```python
from build123d import *

# Parameters (mm, degrees)
SKETCH1_W           = 20
SKETCH1_H           = 40
BOSS_EXTRUDE1_DEPTH = 3
SKETCH4_W           = 8
SKETCH4_H           = 2.4
BOSS_EXTRUDE2_DEPTH = 20
CUT_EXTRUDE1_REACH  = 40.734
SKETCH5_R           = 1.178679728
SKETCH6_R           = 1.5
CUT_EXTRUDE2_DEPTH  = 3


with BuildPart() as part:
    # Sketch1 → Boss-Extrude1 (new body)
    with BuildSketch(Plane(origin=(0, 0, 0), x_dir=(1, 0, 0), z_dir=(0, 1, 0))):
        Rectangle(SKETCH1_W, SKETCH1_H)
    extrude(amount=BOSS_EXTRUDE1_DEPTH)

    # Sketch2 → Loft3 section 0
    with BuildSketch(Plane(origin=(0, 3, 0), x_dir=(1, 0, 0), z_dir=(0, 1, 0))):
        with BuildLine():
            Line((-10, 7.65), (10, 7.65))
            Line((10, 7.65), (10, 1.25))
            Line((10, 1.25), (-10, 1.25))
            Line((-10, 1.25), (-10, 7.65))
        make_face()
    # Sketch3 → Loft3 section 1
    with BuildSketch(Plane(origin=(0, 9, 0), x_dir=(1, 0, 0), z_dir=(0, 1, 0))):
        with BuildLine():
            Line((-4, 3.65), (4, 3.65))
            Line((4, 3.65), (4, 1.25))
            Line((4, 1.25), (-4, 1.25))
            Line((-4, 1.25), (-4, 3.65))
        make_face()
    loft3 = loft()

    # Mirror1: Loft3 across plane
    add(loft3.mirror(Plane(origin=(0, 0, 0), x_dir=(1, 0, 0), z_dir=(0, 0, -1))))

    # Sketch4 → Boss-Extrude2 (add)
    with BuildSketch(Plane(origin=(0, 9, 0), x_dir=(1, 0, 0), z_dir=(0, 1, 0))):
        with Locations((0, 2.45)):
            Rectangle(SKETCH4_W, SKETCH4_H)
        with Locations((0, -2.45)):
            Rectangle(SKETCH4_W, SKETCH4_H)
    extrude(amount=BOSS_EXTRUDE2_DEPTH)

    # Cut-Extrude1: up to this face of the body (flat: up to its plane)
    cut_extrude1_end = Plane(part.part.faces().sort_by_distance((0, 19, -3.65))[0])
    # Sketch5 → Cut-Extrude1 (cut, up to the picked face)
    with BuildSketch(Plane.XY.offset(3.65), mode=Mode.PRIVATE) as cut_extrude1_sk1:
        with BuildLine():
            Line((-4, 29), (-4, 25))
            ThreePointArc((-4, 25), (-2.828427125, 27.828427125), (0, 29))
            Line((0, 29), (-4, 29))
        make_face()
    cut_extrude1_tool1 = split(extrude(cut_extrude1_sk1.sketch, amount=-CUT_EXTRUDE1_REACH, mode=Mode.PRIVATE), bisect_by=cut_extrude1_end, keep=Keep.BOTH, mode=Mode.PRIVATE)
    # Sketch5 → Cut-Extrude1 (cut, up to the picked face)
    with BuildSketch(Plane.XY.offset(3.65), mode=Mode.PRIVATE) as cut_extrude1_sk2:
        with BuildLine():
            Line((4, 29), (0, 29))
            ThreePointArc((0, 29), (2.828427125, 27.828427125), (4, 25))
            Line((4, 25), (4, 29))
        make_face()
    cut_extrude1_tool2 = split(extrude(cut_extrude1_sk2.sketch, amount=-CUT_EXTRUDE1_REACH, mode=Mode.PRIVATE), bisect_by=cut_extrude1_end, keep=Keep.BOTH, mode=Mode.PRIVATE)
    # Sketch5 → Cut-Extrude1 (cut, up to the picked face)
    with BuildSketch(Plane.XY.offset(3.65), mode=Mode.PRIVATE) as cut_extrude1_sk3:
        with Locations((0, 25)):
            Circle(SKETCH5_R)
    cut_extrude1_tool3 = split(extrude(cut_extrude1_sk3.sketch, amount=-CUT_EXTRUDE1_REACH, mode=Mode.PRIVATE), bisect_by=cut_extrude1_end, keep=Keep.BOTH, mode=Mode.PRIVATE)
    add(cut_extrude1_tool1.solids().sort_by(Axis((-3.106528, 28.106528, 3.65), (0, 0, -1)))[0], mode=Mode.SUBTRACT)
    add(cut_extrude1_tool2.solids().sort_by(Axis((3.106528, 28.106528, 3.65), (0, 0, -1)))[0], mode=Mode.SUBTRACT)
    add(cut_extrude1_tool3.solids().sort_by(Axis((0, 25, 3.65), (0, 0, -1)))[0], mode=Mode.SUBTRACT)

    # Sketch6 → Cut-Extrude2 (cut)
    with BuildSketch(Plane(origin=(0, 3, 0), x_dir=(1, 0, 0), z_dir=(0, 1, 0))):
        with Locations(Location((7, 17, 0), (0, 0, 270))):
            Circle(SKETCH6_R)
        with Locations(Location((-7, 17, 0), (0, 0, 270))):
            Circle(SKETCH6_R)
        with Locations(Location((7, -16.463590195, 0), (0, 0, 270))):
            Circle(SKETCH6_R)
        with Locations(Location((-7, -16.463590195, 0), (0, 0, 270))):
            Circle(SKETCH6_R)
    extrude(amount=-CUT_EXTRUDE2_DEPTH, mode=Mode.SUBTRACT)


solid = part.part
```
For this review, take the finished solid that the model builds, in its own axes (mm). A direction names the side the tool comes from. Coordinates: 2 decimals unless noted, no trailing zeros. Loops run counter-clockwise (first coordinate to the right, second up) from the corner with the lowest first, then second, coordinate; pieces in that order, holes last. Notation, with made-up numbers: (62.5, 68.5) - (94.5, 68.5) arc R16 cw to (94.5, 91.5) - close; hole circle Ø10 at (83.5, 17). An arc over 180 degrees is marked (long way). Use one line per item in the form item = value. Start each with the question number.
1) For pin 1 (4 mm diameter, centred on x = 0, y = 25, fed in from +Z); pin 2 (10 mm diameter, centred on x = -3, z = 15.5, fed in from +Y); pin 3 (6.5 mm diameter, centred on x = 0.5, y = 17, fed in from +Z), all flat-tipped, find the tip position at first contact; note any pin that passes through.
2) Take a section at B-B (y = 19). State the section outline as (x, z) points, plus the area to 3 significant figures.
3) Take a section at C-C (x = 7). State how many separate pieces and enclosed holes the cut face has, plus the area to 3 significant figures.
4) To check wall thickness, follow probe 1 along Z at (x, y) = (-0.5, 15.5); probe 2 along Y at (x, z) = (3.75, -16). State the ranges of each line that lie inside material, in increasing order. Write a range as from..to.
5) For faces 4 (the face through (0, 13, 1.25)), 5 (the face through (0, 3, 14)), 6 (the face through (-4, 17, -2)), 7 (the face through (0, 3, -14)), list the 3-axis set-ups (+Z, -Z, +X, -X, +Y, -Y) from which the entire face can be reached by the end or side of a thin tool; tool diameter is ignored.
6) Take a section at D-D (z = -10). State the section outline as (x, y) points, plus the area to 3 significant figures.
7) Draft analysis for pull direction X (two halves, no side actions). For faces 1 (the face through (-4, 17, 2)), 2 (the face through (5.67, 1.52, 17.16)), 3 (the face through (0, 3, 0)), state which applies: released by +X, released by -X, zero draft, split by the parting line, or undercut.
8) Take a section at A-A (z = -17). State the section outline as (x, y) points, plus the area to 3 significant figures.
From the geometry:
q1.pin_1 = 3.65
q1.pin_2 = 3
q1.pin_3 = 3.65
q2.outline = (-4, -3.65) - (4, -3.65) - (4, -1.25) - (-4, -1.25) - close; (-4, 1.25) - (4, 1.25) - (4, 3.65) - (-4, 3.65) - close
q2.area = 38.4 mm2
q3.separate_pieces = 3
q3.enclosed_holes = 0
q3.area = 134 mm2
q4.probe_1 = -3.65..-1.25, 1.25..3.65
q4.probe_2 = 0..3
q5.face_4 = +X, -X, +Y
q5.face_5 = +Z, +X, -X, +Y
q5.face_6 = +Z, -Z, -X, +Y
q5.face_7 = -Z, +X, -X, +Y
q6.outline = (-10, 0) - (10, 0) - (10, 3) - (-10, 3) - close
q6.area = 60.0 mm2
q7.face_1 = released by -X
q7.face_2 = undercut
q7.face_3 = zero draft
q8.outline = (-10, 0) - (-8.5, 0) - (-8.5, 3) - (-10, 3) - close; (-5.5, 0) - (5.5, 0) - (5.5, 3) - (-5.5, 3) - close; (8.5, 0) - (10, 0) - (10, 3) - (8.5, 3) - close
q8.area = 42.0 mm2
